from build123d import *

# Parameters (mm, degrees)
SKETCH1_W                  = 110
SKETCH1_H                  = 10
SKETCH1_R                  = 1.5
BOSS_EXTRUDE1_DEPTH        = 7.7
F_0_8_0_8_DIAMETER_HOLE1_D = 0.8
LPATTERN1_COUNT            = 32
LPATTERN1_PITCH            = 2.54
SKETCH6_W                  = 110
SKETCH6_H                  = 7.7
BOSS_EXTRUDE4_DEPTH        = 0.6
F_1_0MM_DOWEL_HOLE2_D      = 1
F_1_0MM_DOWEL_HOLE2_DEPTH  = 4
F_1_0MM_DOWEL_HOLE2_TIP    = 0.30043031


with BuildPart() as part:
    # Sketch1 → Boss-Extrude1 (new body)
    with BuildSketch(Plane(origin=(0, 0, 0), x_dir=(1, 0, 0), z_dir=(0, 1, 0))):
        Rectangle(SKETCH1_W, SKETCH1_H)
        with Locations((45, 0)):
            Circle(SKETCH1_R, mode=Mode.SUBTRACT)
        with Locations((-45, 0)):
            Circle(SKETCH1_R, mode=Mode.SUBTRACT)
    extrude(amount=BOSS_EXTRUDE1_DEPTH)

    # Ø0.8 (0.8) Diameter Hole1 (through all)
    with Locations(Plane(origin=(-39.37, 7.7, -2.84), x_dir=(0, 0, 1), z_dir=(0, 1, 0))):
        with Locations((0, 0), (2.54, 0), (5.08, 0)):
            f_0_8_0_8_diameter_hole1 = Hole(F_0_8_0_8_DIAMETER_HOLE1_D / 2)

    # LPattern1: Ø0.8 (0.8) Diameter Hole1 ×32
    with Locations(*[(i * LPATTERN1_PITCH, 0, 0) for i in range(1, LPATTERN1_COUNT)]):
        add(f_0_8_0_8_diameter_hole1, mode=Mode.SUBTRACT)

    # Sketch6 → Boss-Extrude4 (add)
    with BuildSketch(Plane(origin=(0, 0, -5), x_dir=(-1, 0, 0), z_dir=(0, 0, -1))):
        with Locations((0, 3.85)):
            Rectangle(SKETCH6_W, SKETCH6_H)
    extrude(amount=BOSS_EXTRUDE4_DEPTH)

    # Ø1.0mm Dowel Hole2
    with Locations(Plane(origin=(-50, 0, -0.3), x_dir=(0, 0, -1), z_dir=(0, -1, 0))):
        with Locations((0, 0), (0, 100)):
            Hole(F_1_0MM_DOWEL_HOLE2_D / 2, depth=F_1_0MM_DOWEL_HOLE2_DEPTH)
            with Locations((0, 0, -(F_1_0MM_DOWEL_HOLE2_DEPTH + F_1_0MM_DOWEL_HOLE2_TIP / 2))):  # 118° drill point
                Cone(0, F_1_0MM_DOWEL_HOLE2_D / 2, F_1_0MM_DOWEL_HOLE2_TIP, mode=Mode.SUBTRACT)


solid = part.part
Input: part model. Units: mm. Frame: model coordinates. Coordinates: 2 decimals unless noted, no trailing zeros. Write each loop counter-clockwise with the first axis right and the second up, starting at its lowest first coordinate (ties: lowest second). Pieces come first, ordered by that corner, then holes. Notation, with made-up numbers: M 43.5,84.5 L 72.5,84.5 A35 ccw 72.5,123.5 Z; hole C 18,16.5 d10. An arc over 180 degrees is marked long. Answer as a JSON object with one key per item and string values. Group by question number.
(1) Ray query, line 1 along X through (y, z) = (1.75, 0.25); line 2 along Z through (x, y) = (39.37, 2.5); line 3 along X through (y, z) = (0.5, 1.25). Return the intervals inside material, ascending. Write a range as [from, to].
(2) Section B-B on y = 1.75. Give the number of separate pieces and of enclosed holes in the cut face, plus the area to 3 significant figures.
(3) Section A-A on x = 45. Output: boundary loops of the cut face in (y, z), plus the area to 3 significant figures.
Result set:
{
 "1": {"line 1": "x = [-55, -46.48], [-43.52, 43.52], [46.48, 55]", "line 2": "z = [-5.6, -3.24], [-2.44, -0.7], [0.1, 1.84], [2.64, 5]", "line 3": "x = [-55, -45.83], [-44.17, 44.17], [45.83, 55]"},
 "2": {"separate pieces": "1", "enclosed holes": "100", "area": "1,100 mm2"},
 "3": {"outline": "M 0,-5.6 L 7.7,-5.6 L 7.7,-1.5 L 0,-1.5 Z; M 0,1.5 L 7.7,1.5 L 7.7,5 L 0,5 Z", "area": "58.5 mm2"}
}
